Source: CAD feature listing. Evaluate the final solid. Frame: model axes, mm. A direction names the side the tool comes from. Give positions to 0.01 mm unless a question says otherwise; leave off trailing zeros. Loops run counter-clockwise (first coordinate to the right, second up) from the corner with the lowest first, then second, coordinate; pieces in that order, holes last. Notation, with made-up numbers: (-3.75, 57.5) -> (33.25, 57.5) arc R4 ccw to (33.25, 62.5) -> close; hole circle Ø5 at (17.5, -20). An arc over 180 degrees is marked (long way). Return JSON: item names as keys, results as strings. Group by question number.
(1) Draft query along Y for faces 3 (the face through (-1, 54, 0)), 4 (the face through (149, -55, 4)), 5 (the face through (-2, -48.5, 9)), 6 (the face through (-1, 51, 7)). Return one class per face: released by +Y, released by -Y, zero draft, split by the parting line, or undercut.
(2) Cut plane A-A on y = 2.5. Return loops of the section in (x, z).
(3) Cut plane B-B on x = -19.5. Return loops of the section in (y, z), then the cut area to 3 significant figures.
(4) Pin query (flat end, axial travel): pin 1 (4.5 mm diameter, centred on x = 22.5, z = 7.5, fed in from -Y); pin 2 (1 mm diameter, centred on y = -27.5, z = 10.5, fed in from -X); pin 3 (5.5 mm diameter, centred on x = -79.5, y = -50.5, fed in from -Z); pin 4 (4 mm diameter, centred on x = -51.5, y = -50.5, fed in from -Z). Return the tip coordinate at first contact, or that it passes through.
(5) Ray query, line 1 (Y direction, x = -49, z = 1); line 2 (X direction, y = 22, z = 2); line 3 (X direction, y = 28, z = 8.25). Return the intervals inside material, ascending. Write a range as from..to.
(6) Access query for faces 1 (the face through (-151, -1, 3)), 2 (the face through (-145, 48, 3)). Directions: +Z, -Z, +X, -X, +Y, -Y. A direction counts if a zero-diameter tool reaches every point of the face in a straight line with its end or side. Return the directions, or none.
```python
from build123d import *

# Parameters (mm, degrees)
SKETCH_W        = 302
SKETCH_H        = 112
SKETCH_W_2      = 287
SKETCH_H_2      = 97
PAD_DEPTH       = 12
FILLET_R        = 5
FILLET001_R     = 5
FILLET002_R     = 5
FILLET003_R     = 5
FILLET004_R     = 5
SKETCH001_W     = 297
SKETCH001_H     = 107
POCKET_DEPTH    = 3
FILLET005_R     = 3
FILLET006_R     = 2
FILLET007_R     = 3
FILLET008_R     = 2
FILLET009_R     = 2
FILLET010_R     = 3
FILLET011_R     = 2
FILLET012_R     = 3
SKETCH002_W     = 80
SKETCH002_H     = 5
POCKET001_DEPTH = 4
SKETCH003_W     = 5
SKETCH003_H     = 32.5
POCKET002_DEPTH = 4
FILLET013_R     = 1
FILLET014_R     = 1
FILLET015_R     = 1
FILLET016_R     = 1
FILLET017_R     = 1
FILLET018_R     = 1
FILLET019_R     = 1
FILLET020_R     = 1
FILLET021_R     = 1
FILLET022_R     = 1
FILLET023_R     = 1
FILLET024_R     = 1
FILLET025_R     = 1
FILLET026_R     = 1
FILLET027_R     = 1
FILLET028_R     = 1
FILLET029_R     = 1
FILLET030_R     = 1
FILLET031_R     = 1
FILLET032_R     = 1
FILLET033_R     = 1
FILLET034_R     = 1
FILLET035_R     = 1
FILLET036_R     = 1
FILLET037_R     = 1
FILLET038_R     = 1
FILLET039_R     = 1
FILLET040_R     = 1
FILLET041_R     = 1
FILLET042_R     = 1
FILLET043_R     = 1
FILLET044_R     = 1
FILLET045_R     = 1
FILLET046_R     = 1
FILLET047_R     = 1
FILLET048_R     = 1
FILLET049_R     = 1
FILLET050_R     = 1
FILLET051_R     = 1
FILLET052_R     = 1


with BuildPart() as part:
    # Sketch → Pad (new body)
    with BuildSketch(Plane.XY):
        Rectangle(SKETCH_W, SKETCH_H)
        Rectangle(SKETCH_W_2, SKETCH_H_2, mode=Mode.SUBTRACT)
    extrude(amount=PAD_DEPTH)

    # Fillet
    fillet_edges = [part.edges().sort_by_distance(p)[0] for p in [
        (151, -56, 6),
    ]]
    fillet(fillet_edges, radius=FILLET_R)

    # Fillet001
    fillet001_edges = [part.edges().sort_by_distance(p)[0] for p in [
        (151, 56, 6),
    ]]
    fillet(fillet001_edges, radius=FILLET001_R)

    # Fillet002
    fillet002_edges = [part.edges().sort_by_distance(p)[0] for p in [
        (-151, 56, 6),
    ]]
    fillet(fillet002_edges, radius=FILLET002_R)

    # Fillet003
    fillet003_edges = [part.edges().sort_by_distance(p)[0] for p in [
        (-151, -56, 6),
    ]]
    fillet(fillet003_edges, radius=FILLET003_R)

    # Fillet004
    fillet004_edges = [part.edges().sort_by_distance(p)[0] for p in [
        (149.535534, -54.535534, 12),
    ]]
    fillet(fillet004_edges, radius=FILLET004_R)

    # Sketch001 (on Face4 of Fillet004) → Pocket (cut)
    with BuildSketch(Plane(origin=(0, 0, 0), x_dir=(1, 0, 0), z_dir=(0, 0, -1))):
        Rectangle(SKETCH001_W, SKETCH001_H)
    extrude(amount=-POCKET_DEPTH, mode=Mode.SUBTRACT)

    # Fillet005
    fillet005_edges = [part.edges().sort_by_distance(p)[0] for p in [
        (148.5, -53.5, 1.5),
    ]]
    fillet(fillet005_edges, radius=FILLET005_R)

    # Fillet006
    fillet006_edges = [part.edges().sort_by_distance(p)[0] for p in [
        (143.5, -48.5, 7.5),
    ]]
    fillet(fillet006_edges, radius=FILLET006_R)

    # Fillet007
    fillet007_edges = [part.edges().sort_by_distance(p)[0] for p in [
        (148.5, 53.5, 1.5),
    ]]
    fillet(fillet007_edges, radius=FILLET007_R)

    # Fillet008
    fillet008_edges = [part.edges().sort_by_distance(p)[0] for p in [
        (143.5, 48.5, 7.5),
    ]]
    fillet(fillet008_edges, radius=FILLET008_R)

    # Fillet009
    fillet009_edges = [part.edges().sort_by_distance(p)[0] for p in [
        (-143.5, 48.5, 7.5),
    ]]
    fillet(fillet009_edges, radius=FILLET009_R)

    # Fillet010
    fillet010_edges = [part.edges().sort_by_distance(p)[0] for p in [
        (-148.5, 53.5, 1.5),
    ]]
    fillet(fillet010_edges, radius=FILLET010_R)

    # Fillet011
    fillet011_edges = [part.edges().sort_by_distance(p)[0] for p in [
        (-143.5, -48.5, 7.5),
    ]]
    fillet(fillet011_edges, radius=FILLET011_R)

    # Fillet012
    fillet012_edges = [part.edges().sort_by_distance(p)[0] for p in [
        (-148.5, -53.5, 1.5),
    ]]
    fillet(fillet012_edges, radius=FILLET012_R)

    # Sketch002 (on Face1 of Fillet012) → Pocket001 (cut)
    with BuildSketch(Plane(origin=(0, 0, 3), x_dir=(1, 0, 0), z_dir=(0, 0, -1))):
        with Locations((-95, 51)):
            Rectangle(SKETCH002_W, SKETCH002_H)
        with Locations((0, 51)):
            Rectangle(SKETCH002_W, SKETCH002_H)
        with Locations((95, 51)):
            Rectangle(SKETCH002_W, SKETCH002_H)
        with Locations((95, -51)):
            Rectangle(SKETCH002_W, SKETCH002_H)
        with Locations((0, -51)):
            Rectangle(SKETCH002_W, SKETCH002_H)
        with Locations((-95, -51)):
            Rectangle(SKETCH002_W, SKETCH002_H)
    extrude(amount=-POCKET001_DEPTH, mode=Mode.SUBTRACT)

    # Sketch003 (on Face1 of Pocket001) → Pocket002 (cut)
    with BuildSketch(Plane(origin=(0, 0, 3), x_dir=(1, 0, 0), z_dir=(0, 0, -1))):
        with Locations((-146, 23.75)):
            Rectangle(SKETCH003_W, SKETCH003_H)
        with Locations((-146, -23.75)):
            Rectangle(SKETCH003_W, SKETCH003_H)
        with Locations((146, 23.75)):
            Rectangle(SKETCH003_W, SKETCH003_H)
        with Locations((146, -23.75)):
            Rectangle(SKETCH003_W, SKETCH003_H)
    extrude(amount=-POCKET002_DEPTH, mode=Mode.SUBTRACT)

    # Fillet013
    fillet013_edges = [part.edges().sort_by_distance(p)[0] for p in [
        (-143.5, -40, 5),
    ]]
    fillet(fillet013_edges, radius=FILLET013_R)

    # Fillet014
    fillet014_edges = [part.edges().sort_by_distance(p)[0] for p in [
        (-135, -48.5, 5),
    ]]
    fillet(fillet014_edges, radius=FILLET014_R)

    # Fillet015
    fillet015_edges = [part.edges().sort_by_distance(p)[0] for p in [
        (-135, -53.5, 5),
    ]]
    fillet(fillet015_edges, radius=FILLET015_R)

    # Fillet016
    fillet016_edges = [part.edges().sort_by_distance(p)[0] for p in [
        (-148.5, -40, 5),
    ]]
    fillet(fillet016_edges, radius=FILLET016_R)

    # Fillet017
    fillet017_edges = [part.edges().sort_by_distance(p)[0] for p in [
        (-148.5, 7.5, 5),
    ]]
    fillet(fillet017_edges, radius=FILLET017_R)

    # Fillet018
    fillet018_edges = [part.edges().sort_by_distance(p)[0] for p in [
        (-143.5, 7.5, 5),
    ]]
    fillet(fillet018_edges, radius=FILLET018_R)

    # Fillet019
    fillet019_edges = [part.edges().sort_by_distance(p)[0] for p in [
        (-148.5, -7.5, 5),
    ]]
    fillet(fillet019_edges, radius=FILLET019_R)

    # Fillet020
    fillet020_edges = [part.edges().sort_by_distance(p)[0] for p in [
        (-143.5, -7.5, 5),
    ]]
    fillet(fillet020_edges, radius=FILLET020_R)

    # Fillet021
    fillet021_edges = [part.edges().sort_by_distance(p)[0] for p in [
        (-148.5, 40, 5),
    ]]
    fillet(fillet021_edges, radius=FILLET021_R)

    # Fillet022
    fillet022_edges = [part.edges().sort_by_distance(p)[0] for p in [
        (-143.5, 40, 5),
    ]]
    fillet(fillet022_edges, radius=FILLET022_R)

    # Fillet023
    fillet023_edges = [part.edges().sort_by_distance(p)[0] for p in [
        (-135, 53.5, 5),
    ]]
    fillet(fillet023_edges, radius=FILLET023_R)

    # Fillet024
    fillet024_edges = [part.edges().sort_by_distance(p)[0] for p in [
        (-135, 48.5, 5),
    ]]
    fillet(fillet024_edges, radius=FILLET024_R)

    # Fillet025
    fillet025_edges = [part.edges().sort_by_distance(p)[0] for p in [
        (-40, 48.5, 5),
    ]]
    fillet(fillet025_edges, radius=FILLET025_R)

    # Fillet026
    fillet026_edges = [part.edges().sort_by_distance(p)[0] for p in [
        (-40, 53.5, 5),
    ]]
    fillet(fillet026_edges, radius=FILLET026_R)

    # Fillet027
    fillet027_edges = [part.edges().sort_by_distance(p)[0] for p in [
        (-55, 48.5, 5),
    ]]
    fillet(fillet027_edges, radius=FILLET027_R)

    # Fillet028
    fillet028_edges = [part.edges().sort_by_distance(p)[0] for p in [
        (-55, 53.5, 5),
    ]]
    fillet(fillet028_edges, radius=FILLET028_R)

    # Fillet029
    fillet029_edges = [part.edges().sort_by_distance(p)[0] for p in [
        (40, 53.5, 5),
    ]]
    fillet(fillet029_edges, radius=FILLET029_R)

    # Fillet030
    fillet030_edges = [part.edges().sort_by_distance(p)[0] for p in [
        (40, 48.5, 5),
    ]]
    fillet(fillet030_edges, radius=FILLET030_R)

    # Fillet031
    fillet031_edges = [part.edges().sort_by_distance(p)[0] for p in [
        (55, 48.5, 5),
    ]]
    fillet(fillet031_edges, radius=FILLET031_R)

    # Fillet032
    fillet032_edges = [part.edges().sort_by_distance(p)[0] for p in [
        (55, 53.5, 5),
    ]]
    fillet(fillet032_edges, radius=FILLET032_R)

    # Fillet033
    fillet033_edges = [part.edges().sort_by_distance(p)[0] for p in [
        (143.5, 40, 5),
    ]]
    fillet(fillet033_edges, radius=FILLET033_R)

    # Fillet034
    fillet034_edges = [part.edges().sort_by_distance(p)[0] for p in [
        (135, 48.5, 5),
    ]]
    fillet(fillet034_edges, radius=FILLET034_R)

    # Fillet035
    fillet035_edges = [part.edges().sort_by_distance(p)[0] for p in [
        (135, 53.5, 5),
    ]]
    fillet(fillet035_edges, radius=FILLET035_R)

    # Fillet036
    fillet036_edges = [part.edges().sort_by_distance(p)[0] for p in [
        (148.5, 40, 5),
    ]]
    fillet(fillet036_edges, radius=FILLET036_R)

    # Fillet037
    fillet037_edges = [part.edges().sort_by_distance(p)[0] for p in [
        (143.5, -7.5, 5),
    ]]
    fillet(fillet037_edges, radius=FILLET037_R)

    # Fillet038
    fillet038_edges = [part.edges().sort_by_distance(p)[0] for p in [
        (148.5, -7.5, 5),
    ]]
    fillet(fillet038_edges, radius=FILLET038_R)

    # Fillet039
    fillet039_edges = [part.edges().sort_by_distance(p)[0] for p in [
        (143.5, -40, 5),
    ]]
    fillet(fillet039_edges, radius=FILLET039_R)

    # Fillet040
    fillet040_edges = [part.edges().sort_by_distance(p)[0] for p in [
        (143.5, 7.5, 5),
    ]]
    fillet(fillet040_edges, radius=FILLET040_R)

    # Fillet041
    fillet041_edges = [part.edges().sort_by_distance(p)[0] for p in [
        (148.5, 7.5, 5),
    ]]
    fillet(fillet041_edges, radius=FILLET041_R)

    # Fillet042
    fillet042_edges = [part.edges().sort_by_distance(p)[0] for p in [
        (148.5, -40, 5),
    ]]
    fillet(fillet042_edges, radius=FILLET042_R)

    # Fillet043
    fillet043_edges = [part.edges().sort_by_distance(p)[0] for p in [
        (135, -48.5, 5),
    ]]
    fillet(fillet043_edges, radius=FILLET043_R)

    # Fillet044
    fillet044_edges = [part.edges().sort_by_distance(p)[0] for p in [
        (135, -53.5, 5),
    ]]
    fillet(fillet044_edges, radius=FILLET044_R)

    # Fillet045
    fillet045_edges = [part.edges().sort_by_distance(p)[0] for p in [
        (40, -53.5, 5),
    ]]
    fillet(fillet045_edges, radius=FILLET045_R)

    # Fillet046
    fillet046_edges = [part.edges().sort_by_distance(p)[0] for p in [
        (40, -48.5, 5),
    ]]
    fillet(fillet046_edges, radius=FILLET046_R)

    # Fillet047
    fillet047_edges = [part.edges().sort_by_distance(p)[0] for p in [
        (55, -48.5, 5),
    ]]
    fillet(fillet047_edges, radius=FILLET047_R)

    # Fillet048
    fillet048_edges = [part.edges().sort_by_distance(p)[0] for p in [
        (55, -53.5, 5),
    ]]
    fillet(fillet048_edges, radius=FILLET048_R)

    # Fillet049
    fillet049_edges = [part.edges().sort_by_distance(p)[0] for p in [
        (-40, -53.5, 5),
    ]]
    fillet(fillet049_edges, radius=FILLET049_R)

    # Fillet050
    fillet050_edges = [part.edges().sort_by_distance(p)[0] for p in [
        (-40, -48.5, 5),
    ]]
    fillet(fillet050_edges, radius=FILLET050_R)

    # Fillet051
    fillet051_edges = [part.edges().sort_by_distance(p)[0] for p in [
        (-55, -48.5, 5),
    ]]
    fillet(fillet051_edges, radius=FILLET051_R)

    # Fillet052
    fillet052_edges = [part.edges().sort_by_distance(p)[0] for p in [
        (-55, -53.5, 5),
    ]]
    fillet(fillet052_edges, radius=FILLET052_R)


solid = part.part
```
Answers:
{
 "1": {"face 3": "zero draft", "face 4": "released by -Y", "face 5": "undercut", "face 6": "undercut"},
 "2": {"outline": "(-151, 0) -> (-148.5, 0) -> (-148.5, 3) -> (-143.5, 3) -> (-143.5, 12) -> (-146, 12) arc R5 ccw to (-151, 7) -> close; (143.5, 3) -> (148.5, 3) -> (148.5, 0) -> (151, 0) -> (151, 7) arc R5 ccw to (146, 12) -> (143.5, 12) -> close"},
 "3": {"outline": "(-56, 0) -> (-53.5, 0) -> (-53.5, 7) -> (-48.5, 7) -> (-48.5, 12) -> (-51, 12) arc R5 ccw to (-56, 7) -> close; (48.5, 7) -> (53.5, 7) -> (53.5, 0) -> (56, 0) -> (56, 7) arc R5 ccw to (51, 12) -> (48.5, 12) -> close", "area": "99.3 mm²"},
 "4": {"pin 1": "y = -56", "pin 2": "x = -150", "pin 3": "z = 7", "pin 4": "z = 3"},
 "5": {"line 1": "-56..-53.5, 53.5..56", "line 2": "-151..-148.5, 148.5..151", "line 3": "-150.84..-143.5, 143.5..150.84"},
 "6": {"face 1": "+Z, -Z, -X, +Y, -Y", "face 2": "-Z"}
}
